Build history of the part. All positions in model axes, mm. Face numbers are marked on the shaded views. Round coordinates to 2 decimals unless told otherwise and drop trailing zeros. Write each loop counter-clockwise with the first axis right and the second up, starting at its lowest first coordinate (ties: lowest second). Pieces come first, ordered by that corner, then holes. Notation, with made-up numbers: (-18, 71.25) -> (15, 71.25) arc R21 ccw to (15, 83.25) -> close; hole circle Ø2 at (76.25, -1). An arc over 180 degrees is marked (long way). Return JSON: item names as keys, results as strings.
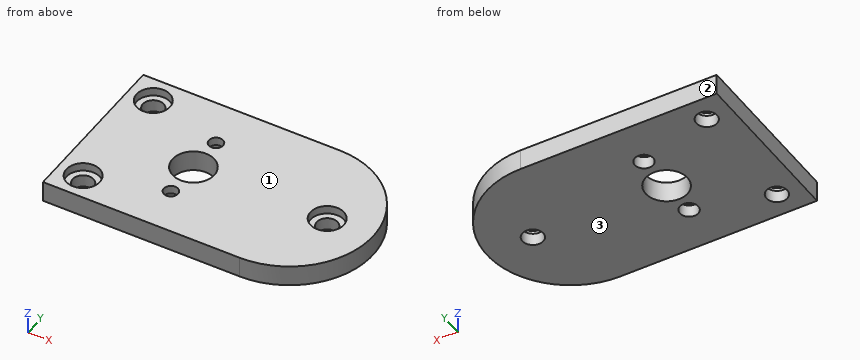
from build123d import *

# Parameters (mm, degrees)
SKETCH_1_R          = 2.5
SKETCH_1_R_2        = 0.85
SKETCH_1_R_3        = 1.25
EXTRUDE_1_DEPTH     = 1.25
CUT_EXTRUDE_START   = 1.25
SKETCH_1_4_R        = 1.1
CUT_EXTRUDE_1_DEPTH = 1.5
CUT_EXTRUDE_START_2 = -1.25
SKETCH_1_5_R        = 2
CUT_EXTRUDE_3_DEPTH = 1
SKETCH_2_W          = 43.696581843
SKETCH_2_H          = 27.281666247
CUT_EXTRUDE_4_DEPTH = 27.804850307


with BuildPart() as part:
    # 草图1 → 凸台-拉伸1 (new, symmetric)
    with BuildSketch(Plane.XY):
        with BuildLine():
            Line((11.5, 10), (-12, 10))
            Line((-12, 10), (-12, -10))
            Line((-12, -10), (11.5, -10))
            ThreePointArc((11.5, -10), (21.5, 0), (11.5, 10))
        make_face()
        Circle(SKETCH_1_R, mode=Mode.SUBTRACT)
        with Locations((0, 4.5)):
            Circle(SKETCH_1_R_2, mode=Mode.SUBTRACT)
        with Locations((0, -4.5)):
            Circle(SKETCH_1_R_2, mode=Mode.SUBTRACT)
        with Locations((-9, 7)):
            Circle(SKETCH_1_R_3, mode=Mode.SUBTRACT)
        with Locations((-9, -7)):
            Circle(SKETCH_1_R_3, mode=Mode.SUBTRACT)
        with Locations((16, 0)):
            Circle(SKETCH_1_R_3, mode=Mode.SUBTRACT)
    extrude(amount=EXTRUDE_1_DEPTH, both=True)

    # 草图1<4> → 切除-拉伸1 (cut)
    with BuildSketch(Plane.XY.offset(CUT_EXTRUDE_START)):
        with Locations((0, 4.5)):
            Circle(SKETCH_1_4_R)
        with Locations((0, -4.5)):
            Circle(SKETCH_1_4_R)
    extrude(amount=-CUT_EXTRUDE_1_DEPTH, mode=Mode.SUBTRACT)

    # 草图1<5> → 切除-拉伸3 (cut)
    with BuildSketch(Plane.XY.offset(CUT_EXTRUDE_START_2)):
        with Locations((-9, 7)):
            Circle(SKETCH_1_5_R)
        with Locations((-9, -7)):
            Circle(SKETCH_1_5_R)
        with Locations((16, 0)):
            Circle(SKETCH_1_5_R)
    extrude(amount=CUT_EXTRUDE_3_DEPTH, mode=Mode.SUBTRACT)


with BuildPart() as body_2:
    # 镜向1: mirrored copy
    add(part.part.mirror(Plane.XY.offset(11.25)))


with BuildPart() as part_1:
    add(part.part)

    # 草图2 → 切除-拉伸4 (cut, through all)
    with BuildSketch(Plane.XY.offset(11.25)):
        with Locations((2.339417989, -1.05223818)):
            Rectangle(SKETCH_2_W, SKETCH_2_H)
    extrude(amount=-CUT_EXTRUDE_4_DEPTH, mode=Mode.SUBTRACT)


solid = body_2.part
Q1. Wall check: L1, parallel to Y at x = -9, z = 21.75; L2, parallel to Y at x = 0, z = 23.3; L3, parallel to Y at x = -9, z = 23.3. Give the ranges that are in metal, low to high.
Verdict:
{"L1": "y = -10 to -8.25, -5.75 to 5.75, 8.25 to 10", "L2": "y = -10 to -5.35, -3.65 to -2.5, 2.5 to 3.65, 5.35 to 10", "L3": "y = -10 to -9, -5 to 5, 9 to 10"}
Q2. Pin check, flat tips, straight feed: pin 1 Ø1 at (y, z) = (-4, 22.5) entering from +X; pin 2 Ø2 at (x, y) = (0, 4.5) entering from -Z; pin 3 Ø2 at (x, y) = (-9, 7) entering from +Z; pin 4 Ø1.5 at (x, z) = (15, 23) entering from +Y. Stop position of each tip, or through.
Verdict:
{"pin 1": "stops at x = 20.87", "pin 2": "stops at z = 22.75", "pin 3": "passes through", "pin 4": "stops at y = 9.61"}
Q3. Saw through at B-B on z = 23.2. List the corners of the cut face in (x, y).
Verdict:
{"outline": "(-12, -10) -> (11.5, -10) arc R10 ccw to (11.5, 10) -> (-12, 10) -> close; hole circle Ø4 at (-9, -7); hole circle Ø4 at (-9, 7); hole circle Ø5 at (0, 0); hole circle Ø1.7 at (0, -4.5); hole circle Ø1.7 at (0, 4.5); hole circle Ø4 at (16, 0)"}
Q4. Saw through at D-D on x = -9. List the corners of the cut face in (y, z).
Verdict:
{"outline": "(-10, 21.25) -> (-8.25, 21.25) -> (-8.25, 22.75) -> (-9, 22.75) -> (-9, 23.75) -> (-10, 23.75) -> close; (-5.75, 21.25) -> (5.75, 21.25) -> (5.75, 22.75) -> (5, 22.75) -> (5, 23.75) -> (-5, 23.75) -> (-5, 22.75) -> (-5.75, 22.75) -> close; (8.25, 21.25) -> (10, 21.25) -> (10, 23.75) -> (9, 23.75) -> (9, 22.75) -> (8.25, 22.75) -> close"}
Q5. Saw through at A-A on x = 2. List the corners of the cut face in (y, z).
Verdict:
{"outline": "(-10, 21.25) -> (-1.5, 21.25) -> (-1.5, 23.75) -> (-10, 23.75) -> close; (1.5, 21.25) -> (10, 21.25) -> (10, 23.75) -> (1.5, 23.75) -> close"}
Q6. Saw through at C-C on y = 6.5. List the corners of the cut face in (x, z), then the cut area to 3 significant figures.
Verdict:
{"outline": "(-12, 21.25) -> (-10.15, 21.25) -> (-10.15, 22.75) -> (-10.94, 22.75) -> (-10.94, 23.75) -> (-12, 23.75) -> close; (-7.85, 21.25) -> (19.1, 21.25) -> (19.1, 23.75) -> (-7.06, 23.75) -> (-7.06, 22.75) -> (-7.85, 22.75) -> close", "area": "70.4 mm²"}
Q7. Two-plate mould, pull along Z, no slides. Class the marked faces 1, 2 and 3: +Z half, -Z half, draft (parallel to the pull), parting line (faces both ways), or undercut.
Verdict:
{"face 1": "+Z half", "face 2": "draft", "face 3": "-Z half"}
